from build123d import *

# Parameters (mm, degrees)
SKETCH1_W                     = 9.144
SKETCH1_H                     = 9.144
BOSS_EXTRUDE1_DEPTH           = 76.2
TAP_DRILL_FOR_8_32_TAP1_D     = 3.4544
TAP_DRILL_FOR_8_32_TAP2_D     = 3.4544
TAP_DRILL_FOR_8_32_TAP3_D     = 3.4544
TAP_DRILL_FOR_8_32_TAP3_DEPTH = 7.62
TAP_DRILL_FOR_8_32_TAP3_TIP   = 1.037806461


with BuildPart() as part:
    # Sketch1 → Boss-Extrude1 (new body)
    with BuildSketch(Plane(origin=(0, 0, 0), x_dir=(1, 0, 0), z_dir=(0, 1, 0))):
        Rectangle(SKETCH1_W, SKETCH1_H)
    extrude(amount=BOSS_EXTRUDE1_DEPTH)

    # Tap Drill for #8-32 Tap1 (through all)
    with Locations(Plane.XY.offset(4.572)):
        with Locations((0, 60.96), (0, 6.35)):
            Hole(TAP_DRILL_FOR_8_32_TAP1_D / 2)

    # Tap Drill for #8-32 Tap2 (through all)
    with Locations(Plane(origin=(4.572, 0, 0), x_dir=(0, 0, -1), z_dir=(1, 0, 0))):
        with Locations((0, 52.07), (0, 15.24)):
            Hole(TAP_DRILL_FOR_8_32_TAP2_D / 2)

    # Tap Drill for #8-32 Tap3
    with Locations(Plane(origin=(0, 76.2, 0), x_dir=(1, 0, 0), z_dir=(0, 1, 0))):
        with Locations((0, 0)):
            Hole(TAP_DRILL_FOR_8_32_TAP3_D / 2, depth=TAP_DRILL_FOR_8_32_TAP3_DEPTH)
            with Locations((0, 0, -(TAP_DRILL_FOR_8_32_TAP3_DEPTH + TAP_DRILL_FOR_8_32_TAP3_TIP / 2))):  # 118° drill point
                Cone(0, TAP_DRILL_FOR_8_32_TAP3_D / 2, TAP_DRILL_FOR_8_32_TAP3_TIP, mode=Mode.SUBTRACT)


solid = part.part
Work out the finished part from the listing and answer in its coordinate system (mm). A direction names the side the tool comes from. Give positions to 0.01 mm unless a question says otherwise; leave off trailing zeros. Write each loop counter-clockwise with the first axis right and the second up, starting at its lowest first coordinate (ties: lowest second). Pieces come first, ordered by that corner, then holes.
Q1. The part is cut by section C-C on x = 3.5. Give the vertices of the cut face in (y, z).
Answer:
outline: (0, -4.57) - (76.2, -4.57) - (76.2, 4.57) - (0, 4.57) - close; hole circle Ø3.45 at (15.24, 0); hole circle Ø3.45 at (52.07, 0)
Q2. For a pull along Z with two mould halves and no side action, classify faces 1 (the face through (0, 38, -4.572)), 2 (the face through (0.225, 8.063, -0.064)), 3 (the face through (-0.064, 16.953, -0.225)) as released by +Z, released by -Z, zero draft, split by the parting line, or undercut.
Answer:
face 1: released by -Z
face 2: zero draft
face 3: undercut
Q3. A tool of negligible diameter and unlimited length cuts with its end or side. For faces 4 (the face through (0, 0, 0)), 5 (the face through (0.225, 72.337, -1.713)), from which of +Z, -Z, +X, -X, +Y, -Y can it reach the whole face along a straight path? Write none if from no direction.
Answer:
face 4: +Z, -Z, +X, -X, -Y
face 5: +Y
Q4. The part is cut by section A-A on y = 52.07. Give the vertices of the cut face in (x, z).
Answer:
outline: (-4.57, -4.57) - (4.57, -4.57) - (4.57, -1.73) - (-4.57, -1.73) - close; (-4.57, 1.73) - (4.57, 1.73) - (4.57, 4.57) - (-4.57, 4.57) - close
Q5. Straight lines are drawn through the part: L1, parallel to Y at x = 0, z = -3.75; L2, parallel to Z at x = 0, y = 72.5; L3, parallel to Y at x = 0.5, z = 1.5. For each, find the intervals that lie inside material, in ascending order.
Answer:
L1: y = 0 to 4.62, 8.08 to 59.23, 62.69 to 76.2
L2: z = -4.57 to -1.73, 1.73 to 4.57
L3: y = 0 to 4.7, 8 to 14.38, 16.1 to 51.21, 52.93 to 59.31, 62.61 to 68.49
Q6. The part is cut by section B-B on z = -3.5. Give the vertices of the cut face in (x, y).
Answer:
outline: (-4.57, 0) - (4.57, 0) - (4.57, 76.2) - (-4.57, 76.2) - close; hole circle Ø3.45 at (0, 6.35); hole circle Ø3.45 at (0, 60.96)
